from build123d import *

# Parameters (mm, degrees)
F0_W     = 100
F0_H     = 100
F1_DEPTH = 100
F2_R     = 5
F3_DEPTH = 100
F5_R     = 10
F6_DEPTH = 25
F7_R     = 5


# Not quite as in the source:
# - a pattern or mirror of a feature is missing from the dataset's text; its kind, count and spacing are read off the source's solid


with BuildPart() as f1:
    # F0 (on Front) → F1 (new body)
    with BuildSketch(Plane.XZ):
        with Locations((50, 50)):
            Rectangle(F0_W, F0_H)
    extrude(amount=F1_DEPTH)

    # F2 (on face) → F3 (cut)
    with BuildSketch(Plane.XZ.offset(100)):
        with Locations((50, 50)):
            Circle(F2_R)
    extrude(amount=-F3_DEPTH, mode=Mode.SUBTRACT)

    # F5 (on face) → F6 (cut)
    with BuildSketch(Plane.XZ.offset(100)):
        with Locations((50, 50)):
            Circle(F5_R)
    f6 = extrude(amount=-F6_DEPTH, mode=Mode.SUBTRACT)

    # F6_copies: F6 across plane
    add(f6.mirror(Plane.ZX.offset(-50)), mode=Mode.SUBTRACT)

    # F7
    f7_edges = [f1.edges().sort_by_distance(p)[0] for p in [
        (0, -50, 100),
        (50, -100, 100),
        (100, -50, 100),
        (50, 0, 100),
        (0, -100, 50),
        (50, -100, 0),
        (100, -100, 50),
        (100, -50, 0),
        (100, 0, 50),
        (50, 0, 0),
        (0, 0, 50),
        (0, -50, 0),
    ]]
    fillet(f7_edges, radius=F7_R)


solid = f1.part
The model under review builds one solid part; all positions refer to its coordinate system, in mm. A direction names the side the tool comes from. Give positions to 0.01 mm unless a question says otherwise; leave off trailing zeros. Write each loop counter-clockwise with the first axis right and the second up, starting at its lowest first coordinate (ties: lowest second). Pieces come first, ordered by that corner, then holes. Notation, with made-up numbers: M -11,64.25 L -7,64.25 A8 ccw -7,74.25 Z; hole C 27.5,8 d6. An arc over 180 degrees is marked long. One line per question, with ' | ' between items. Start each with the question number.
Item 1: Wall thickness on line 1 (Z direction, x = 50, y = -7); line 2 (X direction, y = -80.5, z = 58.5); line 3 (Z direction, x = 50, y = -42): over which ranges is each line inside the solid? List them lowest first. Write a range as from..to.
Item 2: For faces 4 (the cylindrical face through (1, -2, 51)), 5 (the flat face through (45, -25, 48)), list the 3-axis set-ups (+Z, -Z, +X, -X, +Y, -Y) from which the entire face can be reached by the end or side of a thin tool; tool diameter is ignored.
Item 3: For pin 1 (6 mm diameter, centred on x = 53, z = 52.5, fed in from -Y); pin 2 (6 mm diameter, centred on x = 50, z = 50, fed in from +Y), all flat-tipped, find the tip position at first contact; note any pin that passes through.
Item 4: We need section B-B on z = 50. Write out the cut boundary in (x, y), plus the area to 3 significant figures.
Item 5: We need section A-A on x = 50. Write out the cut boundary in (y, z), plus the area to 3 significant figures.
Item 6: Draft analysis for pull direction Z (two halves, no side actions). For faces 1 (the flat face through (49, -49, 0)), 2 (the cylindrical face through (47.83, -87.68, 40.24)), 3 (the cylindrical face through (1, -51, 98)), state which applies: released by +Z, released by -Z, zero draft, split by the parting line, or undercut.
Results found:
1) line 1: z = 0..40, 60..100 | line 2: x = 0..44.73, 55.27..100 | line 3: z = 0..45, 55..100
2) face 4: +Z, -Z, -X, +Y | face 5: +Y
3) pin 1: stops at y = -75 | pin 2: passes through
4) outline: M 0,-95 A5 ccw 5,-100 L 40,-100 L 40,-75 L 45,-75 L 45,-25 L 40,-25 L 40,0 L 5,0 A5 ccw 0,-5 Z; M 55,-75 L 60,-75 L 60,-100 L 95,-100 A5 ccw 100,-95 L 100,-5 A5 ccw 95,0 L 60,0 L 60,-25 L 55,-25 Z | area: 8,480 mm2
5) outline: M -100,5 A5 ccw -95,0 L -5,0 A5 ccw 0,5 L 0,40 L -25,40 L -25,45 L -75,45 L -75,40 L -100,40 Z; M -100,60 L -75,60 L -75,55 L -25,55 L -25,60 L 0,60 L 0,95 A5 ccw -5,100 L -95,100 A5 ccw -100,95 Z | area: 8,480 mm2
6) face 1: released by -Z | face 2: undercut | face 3: released by +Z
